Part model, mm, in its own coordinate system. A direction names the side the tool comes from. Give positions to 0.01 mm unless a question says otherwise; leave off trailing zeros. Write each loop counter-clockwise with the first axis right and the second up, starting at its lowest first coordinate (ties: lowest second). Pieces come first, ordered by that corner, then holes.
Autodesk Inventor part; units mm, degrees
ref_plane "Start plane" through (0, 0, 42) normal (0, 0, 1) x (1, 0, 0)
ref_plane "End plane" through (0, 0, 640) normal (0, 0, 1) x (1, 0, 0)
ref_plane "Work Plane4" through (-1510, -17, 42) normal (0, 0, -1) x (-1, 0, 0)
ref_plane "Start plane" through (0, 0, 42) normal (0, 0, 1) x (1, 0, 0)
ref_plane "End plane" through (0, 0, 640) normal (0, 0, 1) x (1, 0, 0)
sketch "Sketch" plane through (0, 0, 0) normal (0, 0, 1) x (1, 0, 0)
  line L0 (-10, -17) -> (-10, 17)
  line L1 (-7, 20) -> (7, 20)
  line L2 (10, 17) -> (10, -17)
  line L3 (7, -20) -> (-7, -20)
  arc A0 (-10, -17) -> (-7, -20) centre (-7, -17) ccw
  arc A1 (-7, 20) -> (-10, 17) centre (-7, 17) ccw
  arc A2 (10, 17) -> (7, 20) centre (7, 17) ccw
  arc A3 (7, -20) -> (10, -17) centre (7, -17) ccw
  arc A4 (-7, 18) -> (-8, 17) centre (-7, 17) ccw
  line L4 (-7, 18) -> (7, 18)
  arc A5 (8, 17) -> (7, 18) centre (7, 17) ccw
  line L5 (8, 17) -> (8, -17)
  arc A6 (7, -18) -> (8, -17) centre (7, -17) ccw
  line L6 (7, -18) -> (-7, -18)
  arc A7 (-8, -17) -> (-7, -18) centre (-7, -17) ccw
  line L7 (-8, -17) -> (-8, 17)
  line L8 (0, 28.8698) -> (0, -28.8698) construction
  line L9 (-14.8698, 0) -> (14.8698, 0) construction
  dimension "d7" = 3
  dimension "d10" = 40
  dimension "d11" = 20
  dimension "d12" = 2
  dimension "d15" = 20
  dimension "d16" = 10
extrude "Body" add sketch "Sketch" along normal up to surface (598 mm away) from surface at 42
sketch "Sketch3" plane through (0, 0, 0) normal (0, 0, 1) x (1, 0, 0)
  line L0 (0, 0) -> (10, 0)
ref_plane "Work Plane3" through (0, 0, 0) normal (0, -1, 0) x (1, 0, 0)
sketch "Sketch4" plane through (0, 0, 0) normal (0, -1, 0) x (1, 0, 0)
  line L0 (-2, 42) -> (12, 42)
  line L1 (-2, 640) -> (12, 640)
  dimension "d18" = 598
ref_plane "Work Plane4" through (-1510, -17, 42) normal (0, 0, -1) x (-1, 0, 0)
split "Split1" plane through (-1510, -17, 42) removes the side toward (0, 0, -1)
equation "\"d7\" = G_IR"
equation "\"d10\" = G_H"
equation "\"d11\" = G_W"
equation "\"d12\" = G_T"
equation "\"d15\" = 0.5 * d10"
equation "\"d16\" = 0.5 * d11"
equation "\"d3\" = G_L"
equation "\"G_W\" = 20"
equation "\"G_H\" = 40"
equation "\"G_T\" = 2"
equation "\"G_IR\" = 3"
equation "\"G_L\" = d18"
equation "\"G_OFFSET_START\" = -42"
equation "\"G_OFFSET_END\" = 0"
equation "\"d13\" = -G_OFFSET_START"
equation "\"d14\" = G_OFFSET_END + B_L"
equation "\"B_L\" = 640"
properties part number "UNI EN 10305-5 - 40 x 20 x 2  - 598" material "Steel, Mild"
1) Two-plate mould, pull along X, no slides. Class faces 1 (the face through (-8, 0, 337)), 2 (the face through (0, 18, 337)), 3 (the face through (0, -20, 337)), 4 (the face through (-10, 0, 337)): +X half, -X half, draft (parallel to the pull), parting line (faces both ways), or undercut.
Answers follow:
face 1: undercut
face 2: undercut
face 3: draft
face 4: -X half
2) Saw through at A-A, the plane y = 4.5. Write the cut outline in (x, z), then the cut area to 3 significant figures.
Answers follow:
outline: (-10, 42) - (-8, 42) - (-8, 640) - (-10, 640) - close; (8, 42) - (10, 42) - (10, 640) - (8, 640) - close
area: 2,390 mm2
3) Wall check: L1, parallel to Y at x = -7.25, z = 282; L2, parallel to X at y = -2.5, z = 230.5; L3, parallel to Y at x = 8.25, z = 578.5. Give the ranges that are in metal, low to high.
Answers follow:
L1: y = -19.99 to -17.97, 17.97 to 19.99
L2: x = -10 to -8, 8 to 10
L3: y = -19.73 to 19.73
4) Saw through at B-B, the plane x = -1.5. Write the cut outline in (y, z), then the cut area to 3 significant figures.
Answers follow:
outline: (-20, 42) - (-18, 42) - (-18, 640) - (-20, 640) - close; (18, 42) - (20, 42) - (20, 640) - (18, 640) - close
area: 2,390 mm2
5) 3-axis set-ups, long thin cutter, end or side, ignore diameter. For faces 5 (the face through (0, -18, 337)), 6 (the face through (10, 0, 337)): which of +Z, -Z, +X, -X, +Y, -Y reach the whole face in a straight line?
Answers follow:
face 5: +Z, -Z
face 6: +Z, -Z, +X, +Y, -Y
6) Saw through at C-C, the plane z = 150.5. Write the cut outline in (x, y), then the cut area to 3 significant figures.
Answers follow:
outline: (-10, -17) arc R3 ccw to (-7, -20) - (7, -20) arc R3 ccw to (10, -17) - (10, 17) arc R3 ccw to (7, 20) - (-7, 20) arc R3 ccw to (-10, 17) - close; hole (-8, -17) arc R1 ccw to (-7, -18) - (7, -18) arc R1 ccw to (8, -17) - (8, 17) arc R1 ccw to (7, 18) - (-7, 18) arc R1 ccw to (-8, 17) - close
area: 217 mm2
